```python
from build123d import *

# Parameters (mm, degrees)
SKETCH1_W                      = 209.944601778
SKETCH1_H                      = 165.1
BOSS_EXTRUDE1_DEPTH            = 3.302
M5_CLEARANCE_HOLE2_D           = 5.5
M5_CLEARANCE_HOLE2_DEPTH       = 3.302
FILLET1_R                      = 10
BOSS_EXTRUDE2_DEPTH            = 210
F_1_8_0_1250_DOWEL_HOLE1_D     = 3.175
F_1_8_0_1250_DOWEL_HOLE1_DEPTH = 25.4
F_1_8_0_1250_DOWEL_HOLE1_TIP   = 0.953866233
SKETCH25_W                     = 160.0102
SKETCH25_H                     = 1.27
CUT_EXTRUDE1_DEPTH             = 210
SKETCH26_W                     = 160.0102
SKETCH26_H                     = 1.1578
BOSS_EXTRUDE3_DEPTH            = 210
FILLET2_R                      = 2.54


with BuildPart() as part:
    # Sketch1 → Boss-Extrude1 (new body)
    with BuildSketch(Plane(origin=(0, 0, 0), x_dir=(1, 0, 0), z_dir=(0, 1, 0))):
        with Locations((5.037898889, 0)):
            Rectangle(SKETCH1_W, SKETCH1_H)
    extrude(amount=BOSS_EXTRUDE1_DEPTH)

    # M5 Clearance Hole2
    with Locations(Plane(origin=(0, 3.302, 0), x_dir=(1, 0, 0), z_dir=(0, 1, 0))):
        with Locations((71.910199778, -72.55), (-61.834402, -72.55), (71.910199778, 72.55), (-61.834402, 72.55)):
            Hole(M5_CLEARANCE_HOLE2_D / 2, depth=M5_CLEARANCE_HOLE2_DEPTH)

    # Fillet1
    fillet1_edges = [part.edges().sort_by_distance(p)[0] for p in [
        (110.010199778, 1.651, 82.55),
        (-99.934402, 1.651, 82.55),
        (-99.934402, 1.651, -82.55),
        (110.010199778, 1.651, -82.55),
    ]]
    fillet(fillet1_edges, radius=FILLET1_R)

    # Sketch12 → Boss-Extrude2 (add)
    with BuildSketch(Plane.XZ):
        Polygon((85.0051, -59.25), (85.0051, 59.25), (74.9209, 59.25), (74.9209, -49.09), (-64.8451, -49.09), (-64.8451, 59.25), (-75.0051, 59.25), (-75.0051, -59.25), align=None)
    extrude(amount=BOSS_EXTRUDE2_DEPTH)

    # 1/8 (0.1250) Dowel Hole1
    with Locations(Plane(origin=(0, -210, 0), x_dir=(-1, 0, 0), z_dir=(0, -1, 0))):
        with Locations((69.9251, -21.15), (69.9251, 21.15), (36.9051, 54.17), (-56.8949, 54.17), (-79.963, 21.15), (-79.963, -21.15)):
            Hole(F_1_8_0_1250_DOWEL_HOLE1_D / 2, depth=F_1_8_0_1250_DOWEL_HOLE1_DEPTH)
            with Locations((0, 0, -(F_1_8_0_1250_DOWEL_HOLE1_DEPTH + F_1_8_0_1250_DOWEL_HOLE1_TIP / 2))):  # 118° drill point
                Cone(0, F_1_8_0_1250_DOWEL_HOLE1_D / 2, F_1_8_0_1250_DOWEL_HOLE1_TIP, mode=Mode.SUBTRACT)

    # Sketch25 → Cut-Extrude1 (cut)
    with BuildSketch(Plane(origin=(0, -210, 0), x_dir=(-1, 0, 0), z_dir=(0, -1, 0))):
        with Locations((-5, 58.615)):
            Rectangle(SKETCH25_W, SKETCH25_H)
    extrude(amount=-CUT_EXTRUDE1_DEPTH, mode=Mode.SUBTRACT)

    # Sketch26 → Boss-Extrude3 (add)
    with BuildSketch(Plane(origin=(0, -210, 0), x_dir=(-1, 0, 0), z_dir=(0, -1, 0))):
        with Locations((-5, 58.5589)):
            Rectangle(SKETCH26_W, SKETCH26_H)
    extrude(amount=-BOSS_EXTRUDE3_DEPTH)

    # Fillet2
    fillet2_edges = [part.edges().sort_by_distance(p)[0] for p in [
        (-75.0051, -105, -59.1378),
        (85.0051, -105, -59.1378),
        (74.9209, -105, 59.25),
        (-64.8451, -105, 59.25),
        (-75.0051, -105, 59.25),
        (85.0051, -105, 59.25),
    ]]
    fillet(fillet2_edges, radius=FILLET2_R)


solid = part.part
```
Geometry check sheet. Reference: the model listing, model coordinates, mm. A direction names the side the tool comes from. Coordinates: 2 decimals unless noted, no trailing zeros. Loops run counter-clockwise (first coordinate to the right, second up) from the corner with the lowest first, then second, coordinate; pieces in that order, holes last.
Item 1: Sectioned sample at A-A, the plane y = -175.5. Record the boundary of the cut face in (x, z).
Item 2: Thickness scan on line 1 (X direction, y = 1.6, z = 72.55); line 2 (X direction, y = -202, z = 21); line 3 (X direction, y = -198.75, z = -21.15). Record the ranges inside material, lowest first.
Item 3: Release check for a two-part mould opening along Z. For faces 1 (the face through (70.64, 1.63, -70.11)), 2 (the face through (-64.845, -104, 3)), 3 (the face through (6, -104, -49.09)), 4 (the face through (-61.238, 1.628, -69.865)) record: released by +Z, released by -Z, zero draft, split by the parting line, or undercut.
Item 4: Access from +Z, -Z, +X, -X, +Y, -Y to the whole of each face (thin tool, end or side, straight path). Record for faces 5 (the face through (6, -106, -59.138)), 6 (the face through (-59.8, 1.6, 70.7)), 7 (the face through (-75.005, -106, 1)), 8 (the face through (74.921, -104, 5)), 9 (the face through (85.005, -106, 1)).
Item 5: Sectioned sample at D-D, the plane x = 93.5. Record the boundary of the cut face in (y, z).
Item 6: Sectioned sample at C-C, the plane z = 46. Record the boundary of the cut face in (x, y), then the cut area to 3 significant figures.
Item 7: Go/stop test with flat-tipped pins: pin 1 Ø3 at (y, z) = (-93, -59) entering from -X; pin 2 Ø3 at (x, y) = (-41.5, -70.5) entering from -Z; pin 3 Ø7 at (x, z) = (-61.83, 72.55) entering from -Y; pin 4 Ø3.5 at (x, z) = (71.91, 72.55) entering from +Y. Record where each tip stops, or that it passes through.
Item 8: Sectioned sample at B-B, the plane x = 51. Record the boundary of the cut face in (y, z), then the cut area to 3 significant figures.
Check result:
1. outline: (-75.01, -56.6) arc R2.54 ccw to (-72.47, -59.14) - (82.47, -59.14) arc R2.54 ccw to (85.01, -56.6) - (85.01, 56.71) arc R2.54 ccw to (82.47, 59.25) - (77.46, 59.25) arc R2.54 ccw to (74.92, 56.71) - (74.92, -49.09) - (-64.85, -49.09) - (-64.85, 56.71) arc R2.54 ccw to (-67.39, 59.25) - (-72.47, 59.25) arc R2.54 ccw to (-75.01, 56.71) - close
2. line 1: x = -99.93 to -64.58, -59.08 to 69.16, 74.66 to 110.01
2. line 2: x = -75.01 to -71.51, -68.34 to -64.85, 74.92 to 78.38, 81.54 to 85.01
2. line 3: x = -75.01 to -71.51, -68.34 to -64.85, 74.92 to 78.38, 81.55 to 85.01
3. face 1: undercut
3. face 2: zero draft
3. face 3: released by +Z
3. face 4: undercut
4. face 5: -Z, +X, -X, -Y
4. face 6: +Y, -Y
4. face 7: +Z, -Z, -X, -Y
4. face 8: +Z, -Y
4. face 9: +Z, -Z, +X, -Y
5. outline: (0, -82.55) - (3.3, -82.55) - (3.3, 82.55) - (0, 82.55) - close
6. outline: (-99.93, 0) - (-75.01, 0) - (-75.01, -210) - (-64.85, -210) - (-64.85, 0) - (74.92, 0) - (74.92, -210) - (85.01, -210) - (85.01, 0) - (110.01, 0) - (110.01, 3.3) - (-99.93, 3.3) - close
6. area: 4,940 mm2
7. pin 1: stops at x = -74.84
7. pin 2: stops at z = -59.14
7. pin 3: stops at y = 0
7. pin 4: passes through
8. outline: (-210, -59.14) - (0, -59.14) - (0, -82.55) - (3.3, -82.55) - (3.3, 82.55) - (0, 82.55) - (0, -49.09) - (-210, -49.09) - close
8. area: 2,660 mm2
